Autodesk Inventor part; units mm, degrees
ref_plane "YZ Plane" through (0, 0, 0) normal (1, 0, 0) x (0, 1, 0)
ref_plane "XZ Plane" through (0, 0, 0) normal (0, 1, 0) x (-1, 0, 0)
ref_plane "XY Plane" through (0, 0, 0) normal (0, 0, 1) x (1, 0, 0)
sketch "Sketch2" plane through (0, 0, 0) normal (0, 0, 1) x (1, 0, 0)
  line L0 (0, 0) -> (-32.5, 0)
  line L1 (-32.5, 0) -> (-32.5, 25)
  line L2 (-32.5, 25) -> (-12.5, 25)
  line L3 (-12.5, 25) -> (-12.5, 22.5)
  line L4 (-12.5, 22.5) -> (12.5, 22.5)
  line L5 (12.5, 22.5) -> (12.5, 25)
  line L6 (12.5, 25) -> (32.5, 25)
  line L7 (32.5, 25) -> (32.5, 0)
  line L8 (32.5, 0) -> (0, 0)
  line L9 (-12.5, 22.5) -> (0, 10)
  line L10 (0, 10) -> (12.5, 22.5)
  line L11 (-45.5, 0) -> (45.5, 0)
  point P0 (0, 22.5)
  dimension "d1" = 20
  dimension "d2" = 65
  dimension "d4" = 25
  dimension "d5" = 45
  dimension "d6" = 45
  dimension "d7" = 5
revolve "Revolution1" add sketch "Sketch2" angle 360 about axis through (-10, 0, 0) along (1, 0, 0) contours L0 L1 L2 L3 L9 L10 L5 L6 L7 L8
fillet "Fillet1" radius 1 1 edges at (0, -10, 0)
sketch "Sketch3" plane through (-32.5, 0, 0) normal (-1, 0, 0) x (0, 0, 1)
  circle A0 centre (0, 0) radius 5.02
  dimension "d10" = 10.04
extrude "Extrusion1" cut sketch "Sketch3" against normal through all
sketch "Sketch5" plane through (0, 0, 0) normal (0, 1, 0) x (-1, 0, 0)
  line L0 (-32.5, 25) -> (-32.5, -25)
  line L1 (-32.5, 0) -> (32.6883, 0)
  line L2 (-12.5, 25) -> (-32.5, 25)
  line L3 (-22.5, 25) -> (-22.5, -25)
  line L4 (-12.5, -25) -> (-32.5, -25)
  line L5 (32.5, 25) -> (12.5, 25)
  line L6 (22.5, 25) -> (22.5, -25)
  line L7 (32.5, -25) -> (12.5, -25)
  circle A0 centre (-22.5, 0) radius 2.75
  point P0 (0, 0)
  dimension "d13" = 5.5
extrude "Extrusion2" cut sketch "Sketch5" against normal through all contours A0 L3 L1 | L1 L3 A0 | A0 L1 L3 | L1 A0 L3
properties part number "guideWheel"
Design review of the part built by this model. Coordinates are the model's own, in mm. A direction names the side the tool comes from. Give positions to 0.01 mm unless a question says otherwise; leave off trailing zeros. Write each loop counter-clockwise with the first axis right and the second up, starting at its lowest first coordinate (ties: lowest second). Pieces come first, ordered by that corner, then holes. Notation, with made-up numbers: M 35.25,21 L 74.25,21 A11 ccw 74.25,41 Z; hole C 47,33 d10. An arc over 180 degrees is marked long. Answer as a JSON object with one key per item and string values. Group by question number.
1) Tool access review of faces 1 (the face through (-22.36, 23.846, 7.509)), 2 (the face through (1.44, -2.48, -11.17)): name each direction out of +Z, -Z, +X, -X, +Y, -Y from which nothing blocks a thin tool from reaching the whole face with its end or side.
2) We need section D-D (x = 21.5). Give the boundary of the cut face in (y, z), and give its area (3 significant figures).
3) For line 1 along X through (y, z) = (-22.5, 1); line 2 along X through (y, z) = (-21, 1); line 3 along X through (y, z) = (-8.5, 0), list the stretches that pass through material, from the lowest coordinate up.
4) We need section A-A (x = 5). Give the boundary of the cut face in (y, z).
5) We need section C-C (x = -13.5). Give the boundary of the cut face in (y, z).
6) Mouldability with a two-part tool opening along Z and no side actions: class faces 3 (the face through (22.64, 23.846, 7.509)), 4 (the face through (25.247, -14.454, 0.121)), 5 (the face through (-0.455, 4.977, -0.654)), 6 (the face through (-12.5, -22.34, 3.82)) as released by +Z, released by -Z, zero draft, split by the parting line, or undercut.
7) Clearance check with flat-ended pins moving along their axes: pin 1 Ø3 at (x, y) = (-10.5, -13.5) entering from -Z; pin 2 Ø1 at (x, y) = (18, -12.5) entering from +Z; pin 3 Ø5 at (x, y) = (-4.5, 9) entering from +Z. State where each tip first meets the part, or that it passes through.
8) We need section B-B (z = 0). Count the separate pieces of the cut face and the enclosed holes in it, and give its area (3 significant figures).
Answer key:
{
 "1": {"face 1": "+X, -X", "face 2": "none"},
 "2": {"outline": "M -24.87,-2.56 A25 ccw long -24.87,2.56 L -4.32,2.56 A5.02 cw long -4.32,-2.56 Z", "area": "1,780 mm²"},
 "3": {"line 1": "x = -32.5 to -12.5, 12.5 to 19.94, 25.06 to 32.5", "line 2": "x = -32.5 to -11.02, 11.02 to 19.94, 25.06 to 32.5", "line 3": "x = -32.5 to 19.75, 25.25 to 32.5"},
 "4": {"outline": "C 0,0 d30; hole C 0,0 d10.04"},
 "5": {"outline": "C 0,0 d50; hole C 0,0 d10.04"},
 "6": {"face 3": "split by the parting line", "face 4": "undercut", "face 5": "undercut", "face 6": "zero draft"},
 "7": {"pin 1": "stops at z = -17.68", "pin 2": "stops at z = 21.93", "pin 3": "stops at z = 14.76"},
 "8": {"separate pieces": "3", "enclosed holes": "0", "area": "2,050 mm²"}
}
